CAD build for the part. Positions are in the model's coordinates, mm. A direction names the side the tool comes from. Give positions to 0.01 mm unless a question says otherwise; leave off trailing zeros. Loops run counter-clockwise (first coordinate to the right, second up) from the corner with the lowest first, then second, coordinate; pieces in that order, holes last.
Item 1: Saw through at D-D on y = 5.5. Give the cut face in (x, z).
Item 2: Saw through at C-C on z = 71.5. Give the cut face in (x, y), plus the area to 3 significant figures.
Item 3: Saw through at A-A on x = 1.75. Give the cut face in (y, z).
Item 4: Probe probe 1 along X at (y, z) = (2.25, 75.5); probe 2 along X at (y, z) = (-4.5, 54). List the from-to ranges inside material, lowest first.
Item 5: Which spindle directions (+Z, -Z, +X, -X, +Y, -Y) get a long thin tool onto all of the face, cutting with end or side? Do faces 1 (the flat face through (-4.699, 0, 45)), 2 (the cylindrical face through (5.79, -5.75, 45.08)). Say none if no direction does.
Item 6: Drop a flat-ended pin along its axis: P1, Ø3, axis at x = -4, y = -1, coming from the -Z side. Give the stop position or say it passes through.
Autodesk Inventor part; units mm, degrees
ref_plane "Start plane" through (0, 0, 0) normal (0, 0, 1) x (1, 0, 0)
ref_plane "End plane" through (0, 0, 91.44) normal (0, 0, 1) x (1, 0, 0)
ref_plane "YZ Plane" through (0, 0, 0) normal (1, 0, 0) x (0, 1, 0)
ref_plane "Start plane" through (0, 0, 0) normal (0, 0, 1) x (1, 0, 0)
ref_plane "End plane" through (0, 0, 91.44) normal (0, 0, 1) x (1, 0, 0)
sketch "Sketch" plane through (0, 0, 0) normal (0, 0, 1) x (1, 0, 0)
  line L0 (-6.35, -4.3688) -> (-6.35, 4.3688)
  line L1 (-4.3688, 6.35) -> (4.3688, 6.35)
  line L2 (6.35, 4.3688) -> (6.35, -4.3688)
  line L3 (4.3688, -6.35) -> (-4.3688, -6.35)
  arc A0 (-6.35, -4.3688) -> (-4.3688, -6.35) centre (-4.3688, -4.3688) ccw
  arc A1 (-4.3688, 6.35) -> (-6.35, 4.3688) centre (-4.3688, 4.3688) ccw
  arc A2 (6.35, 4.3688) -> (4.3688, 6.35) centre (4.3688, 4.3688) ccw
  arc A3 (4.3688, -6.35) -> (6.35, -4.3688) centre (4.3688, -4.3688) ccw
  arc A4 (-4.3688, 4.699) -> (-4.699, 4.3688) centre (-4.3688, 4.3688) ccw
  line L4 (-4.3688, 4.699) -> (4.3688, 4.699)
  arc A5 (4.699, 4.3688) -> (4.3688, 4.699) centre (4.3688, 4.3688) ccw
  line L5 (4.699, 4.3688) -> (4.699, -4.3688)
  arc A6 (4.3688, -4.699) -> (4.699, -4.3688) centre (4.3688, -4.3688) ccw
  line L6 (4.3688, -4.699) -> (-4.3688, -4.699)
  arc A7 (-4.699, -4.3688) -> (-4.3688, -4.699) centre (-4.3688, -4.3688) ccw
  line L7 (-4.699, -4.3688) -> (-4.699, 4.3688)
  line L8 (0, 9.4644) -> (0, -9.4644) construction
  line L9 (-10.1124, 0) -> (13.3521, 0) construction
  dimension "d10" = 12.7
  dimension "d11" = 12.7
  dimension "d12" = 1.651
  dimension "d15" = 6.35
  dimension "d16" = 6.35
  dimension "d17" = 1.9812
extrude "Body" add sketch "Sketch" along normal up to surface (91.44 mm away) from surface at 0
sketch "Sketch3" plane through (0, 0, 0) normal (0, 0, 1) x (1, 0, 0)
  line L0 (0, 0) -> (10, 0)
ref_plane "Work Plane3" through (0, 0, 0) normal (0, -1, 0) x (1, 0, 0)
sketch "Sketch4" plane through (0, 0, 0) normal (0, -1, 0) x (1, 0, 0)
  line L0 (-2, 0) -> (12, 0)
  line L1 (-2, 91.44) -> (12, 91.44)
  dimension "d19" = 91.44
sketch "Sketch5" plane through (-6.35, 4.3688, 0) normal (-1, 0, 0) x (0, 0, 1)
  point P0 (0, -4.3688)
equation "\"d10\" = G_H"
equation "\"d11\" = G_W"
equation "\"d12\" = G_T"
equation "\"d15\" = 0.5 * d10"
equation "\"d16\" = 0.5 * d11"
equation "\"d17\" = G_IR"
equation "\"d3\" = G_L"
equation "\"G_W\" = 12.7"
equation "\"G_H\" = 12.7"
equation "\"G_T\" = 1.651"
equation "\"G_IR\" = 1.2 * G_T"
equation "\"G_L\" = d19"
equation "\"G_OFFSET_START\" = 0"
equation "\"G_OFFSET_END\" = 0"
equation "\"d14\" = G_OFFSET_END + B_L"
equation "\"B_L\" = 91.44"
properties part number "ASTM A513 - 1/2 x 1/2 x 13/200 - 3.6" material "Steel, Mild"
Results below:
1. outline: (-6, 0) - (6, 0) - (6, 91.44) - (-6, 91.44) - close
2. outline: (-6.35, -4.37) arc R1.98 ccw to (-4.37, -6.35) - (4.37, -6.35) arc R1.98 ccw to (6.35, -4.37) - (6.35, 4.37) arc R1.98 ccw to (4.37, 6.35) - (-4.37, 6.35) arc R1.98 ccw to (-6.35, 4.37) - close; hole (-4.7, -4.37) arc R0.33 ccw to (-4.37, -4.7) - (4.37, -4.7) arc R0.33 ccw to (4.7, -4.37) - (4.7, 4.37) arc R0.33 ccw to (4.37, 4.7) - (-4.37, 4.7) arc R0.33 ccw to (-4.7, 4.37) - close
2. area: 69.7 mm2
3. outline: (-6.35, 0) - (-4.7, 0) - (-4.7, 91.44) - (-6.35, 91.44) - close; (4.7, 0) - (6.35, 0) - (6.35, 91.44) - (4.7, 91.44) - close
4. probe 1: x = -6.35 to -4.7, 4.7 to 6.35
4. probe 2: x = -6.35 to -4.67, 4.67 to 6.35
5. face 1: +Z, -Z
5. face 2: +Z, -Z, +X, -Y
6. P1: stops at z = 0
